```python
from build123d import *

# Parameters (mm, degrees)
ESBO_O2_R                   = 9.5
RESSALTO_EXTRUS_O3_DEPTH    = 9
RESSALTO_EXTRUS_O3_TAPER    = 25
CORTE_EXTRUS_O1_DEPTH       = 8
CORTE_EXTRUS_O4_DEPTH       = 10
CORTE_EXTRUS_O4_DEPTH_BACK  = 8
ESBO_O12_R                  = 1.55
CORTE_EXTRUS_O5_DEPTH       = 5
CORTE_EXTRUS_O5_DEPTH_BACK  = 8
ESBO_O20_R                  = 2.65
CORTE_EXTRUS_O6_DEPTH       = 9.8
CORTE_EXTRUS_O6_DEPTH_BACK  = 10
ESBO_O36_R                  = 1.6
CORTE_EXTRUS_O8_DEPTH       = 10
RESSALTO_EXTRUS_O4_START    = 10
ESBO_O36_3_R                = 9.5
ESBO_O36_3_R_2              = 4
ESBO_O36_3_R_3              = 1.6
RESSALTO_EXTRUS_O4_DEPTH    = 10
CORTE_EXTRUS_O10_DEPTH      = 10
CORTE_EXTRUS_O10_DEPTH_BACK = 9.9
CORTE_EXTRUS_O11_DEPTH      = 9.9
CORTE_EXTRUS_O11_DEPTH_BACK = 9.9


with BuildPart() as part:
    # Esbo_o2 → Ressalto-extrus_o3 (new body)
    with BuildSketch(Plane.XY.offset(10)):
        Circle(ESBO_O2_R)
    extrude(amount=RESSALTO_EXTRUS_O3_DEPTH, taper=RESSALTO_EXTRUS_O3_TAPER)

    # Esbo_o8 → Corte-extrus_o1 (cut)
    with BuildSketch(Plane.XY.offset(19)):
        with BuildLine():
            ThreePointArc((-1.687453703, 1.25), (-1.875499933, -0.944722181), (0, -2.1))
            Line((0, -2.1), (0, 1.25))
            Line((0, 1.25), (-1.687453703, 1.25))
        make_face()
        with BuildLine():
            Line((0, 1.25), (0, -2.1))
            ThreePointArc((0, -2.1), (1.48492424, -1.48492424), (2.1, 0))
            ThreePointArc((2.1, 0), (1.994198182, 0.65815926), (1.687453703, 1.25))
            Line((1.687453703, 1.25), (0, 1.25))
        make_face()
    extrude(amount=-CORTE_EXTRUS_O1_DEPTH, mode=Mode.SUBTRACT)

    # Esbo_o12 → Corte-extrus_o4 (cut, two sides: drawn at the far end of the back side and taken through both)
    with BuildSketch(Plane(origin=(0, 9.25, 0), x_dir=(-1, 0, 0), z_dir=(0, -1, 0)).offset(-CORTE_EXTRUS_O4_DEPTH_BACK)):
        with Locations(Location((0.013800593, -14.999427624, 0), (0, 0, 335.62815521))):
            Circle(ESBO_O12_R)
    extrude(amount=CORTE_EXTRUS_O4_DEPTH + CORTE_EXTRUS_O4_DEPTH_BACK, mode=Mode.SUBTRACT)

    # Esbo_o20 → Corte-extrus_o5 (cut, two sides: drawn at the far end of the back side and taken through both)
    with BuildSketch(Plane(origin=(0, 9.25, 0), x_dir=(-1, 0, 0), z_dir=(0, -1, 0)).offset(-CORTE_EXTRUS_O5_DEPTH_BACK)):
        with Locations(Location((0.013800593, -14.999427624, 0), (0, 0, 10.257774757))):
            Circle(ESBO_O20_R)
    extrude(amount=CORTE_EXTRUS_O5_DEPTH + CORTE_EXTRUS_O5_DEPTH_BACK, mode=Mode.SUBTRACT)

    # Esbo_o25 → Corte-extrus_o6 (cut, two sides: drawn at the far end of the back side and taken through both)
    with BuildSketch(Plane(origin=(0, 0, 20), x_dir=(-1, 0, 0), z_dir=(0, 0, -1)).offset(-CORTE_EXTRUS_O6_DEPTH_BACK)):
        Polygon((7.134775628, 3.121360799), (4.053715986, 2.352982757), (3.178621068, -0.699482185), (5.384585793, -2.983569084), (8.465645436, -2.215191043), (9.340740353, 0.837273899), align=None)
        Polygon((-5.961169976, 3.129376222), (-8.940704294, 2.0313286), (-9.479534318, -1.098047621), (-7.038830024, -3.129376222), (-4.059295706, -2.0313286), (-3.520465682, 1.098047621), align=None)
    extrude(amount=CORTE_EXTRUS_O6_DEPTH + CORTE_EXTRUS_O6_DEPTH_BACK, mode=Mode.SUBTRACT)

    # Esbo_o36 → Corte-extrus_o8 (cut)
    with BuildSketch(Plane(origin=(0, 0, 10), x_dir=(-1, 0, 0), z_dir=(0, 0, -1))):
        with Locations((-6.5, 0)):
            Circle(ESBO_O36_R)
        with Locations((6.5, 0)):
            Circle(ESBO_O36_R)
    extrude(amount=-CORTE_EXTRUS_O8_DEPTH, mode=Mode.SUBTRACT)

    # Esbo_o36_3 → Ressalto-extrus_o4 (add)
    # profile 1 of 2: a face of its own
    with BuildSketch(Plane(origin=(0, 0, 10), x_dir=(-1, 0, 0), z_dir=(0, 0, -1)).offset(RESSALTO_EXTRUS_O4_START)):
        Circle(ESBO_O36_3_R)
        Circle(ESBO_O36_3_R_2, mode=Mode.SUBTRACT)
        with Locations((6.5, 0)):
            Circle(ESBO_O36_3_R_3, mode=Mode.SUBTRACT)
        with Locations((-6.5, 0)):
            Circle(ESBO_O36_3_R_3, mode=Mode.SUBTRACT)
    # profile 2 of 2: a face of its own
    with BuildSketch(Plane(origin=(0, 0, 10), x_dir=(-1, 0, 0), z_dir=(0, 0, -1)).offset(RESSALTO_EXTRUS_O4_START)):
        with BuildLine():
            Line((0.99979998, 0.98), (-0.99979998, 0.98))
            ThreePointArc((-0.99979998, 0.98), (-0.529282546, -1.296094127), (1.4, 0))
            ThreePointArc((1.4, 0), (1.296094127, 0.529282546), (0.99979998, 0.98))
        make_face()
    extrude(amount=-RESSALTO_EXTRUS_O4_DEPTH)

    # Esbo_o49 → Corte-extrus_o10 (cut, two sides: drawn at the far end of the back side and taken through both)
    with BuildSketch(Plane(origin=(0, 0, 20), x_dir=(-1, 0, 0), z_dir=(0, 0, -1)).offset(-CORTE_EXTRUS_O10_DEPTH_BACK)):
        with BuildLine():
            Line((8.371054684, 4.491708302), (4.673014458, 2.507428111))
            Line((4.673014458, 2.507428111), (4.053715986, 2.352982757))
            Line((4.053715986, 2.352982757), (3.178621068, -0.699482185))
            Line((3.178621068, -0.699482185), (4.760398724, -2.337277014))
            Line((4.760398724, -2.337277014), (7.818914356, -5.395792647))
            ThreePointArc((7.818914356, -5.395792647), (9.069996868, -2.825801976), (9.5, 0))
            ThreePointArc((9.5, 0), (9.213441797, 2.31570513), (8.371054684, 4.491708302))
        make_face()
    extrude(amount=CORTE_EXTRUS_O10_DEPTH + CORTE_EXTRUS_O10_DEPTH_BACK, mode=Mode.SUBTRACT)

    # Esbo_o49_4 → Corte-extrus_o11 (cut, two sides: drawn at the far end of the back side and taken through both)
    with BuildSketch(Plane(origin=(0, 0, 20), x_dir=(-1, 0, 0), z_dir=(0, 0, -1)).offset(-CORTE_EXTRUS_O11_DEPTH_BACK)):
        with BuildLine():
            Line((-3.520465682, 1.098047621), (-4.830623712, 2.188454798))
            Line((-4.830623712, 2.188454798), (-8.141518287, 4.89547546))
            ThreePointArc((-8.141518287, 4.89547546), (-9.48963755, 0.443597976), (-8.562700205, -4.114628197))
            Line((-8.562700205, -4.114628197), (-4.779997666, -2.296928855))
            Line((-4.779997666, -2.296928855), (-4.059295706, -2.0313286))
            Line((-4.059295706, -2.0313286), (-3.520465682, 1.098047621))
        make_face()
    extrude(amount=CORTE_EXTRUS_O11_DEPTH + CORTE_EXTRUS_O11_DEPTH_BACK, mode=Mode.SUBTRACT)


solid = part.part
```
Verification items for the finished model (mm, model axes). A direction names the side the tool comes from. Give positions to 0.01 mm unless a question says otherwise; leave off trailing zeros. Write each loop counter-clockwise with the first axis right and the second up, starting at its lowest first coordinate (ties: lowest second). Pieces come first, ordered by that corner, then holes. Notation, with made-up numbers: (49.25, 52.25) - (96.25, 52.25) arc R20 cw to (96.25, 85.25) - close; hole circle Ø10 at (25.5, 12). An arc over 180 degrees is marked (long way). Put each result on its own line as item: value.
Q1. Section check A-A on z = 6. Record the cut outline in (x, y).
Result:
outline: circle Ø19 at (0, 0); (-1, 0.98) arc R1.4 ccw (long way) to (1, 0.98) - close; hole circle Ø3.2 at (-6.5, 0); hole circle Ø8 at (0, 0); hole circle Ø3.2 at (6.5, 0)
Q2. Mould release check, pull along X, two halves, no side actions. Record for faces 6 (the face through (-5.726, 3.073, 12.563)), 7 (the face through (5.85, -2.81, 12.63)), 8 (the face through (-8, -1, 10)), 9 (the face through (8.1, 0.07, 4.98)): released by +X, released by -X, zero draft, split by the parting line, or undercut.
Result:
face 6: released by -X
face 7: released by +X
face 8: zero draft
face 9: undercut
Q3. Scan lines: probe 1 along Y at (x, z) = (0.25, 6.5); probe 2 along X at (y, z) = (-0.25, 8.75); probe 3 along Z at (x, y) = (-2.25, 0.5). Record each from-to range of solid material in increasing order. Write a range as from..to.
Result:
probe 1: -9.5..-3.99, -1.38..0.98, 3.99..9.5
probe 2: -9.5..-8.08, -4.92..-3.99, -1.38..1.38, 3.99..4.92, 8.08..9.5
probe 3: 10..19
Q4. Set-up check for faces 1 (the face through (0.794, 5.895, 12.475)), 2 (the face through (-6.268, -3.845, 12.034)), 3 (the face through (2, 0, 10)), 4 (the face through (8, 1, 10.1)), 5 (the face through (0, 0, 11)): record each of +Z, -Z, +X, -X, +Y, -Y from which the full face is reachable in a straight line by a thin tool's end or side.
Result:
face 1: +Y
face 2: +Z, -X
face 3: -Z
face 4: +Z, +X
face 5: +Z
Q5. Depth check by flat-ended pin: P1, Ø1.6, axis at x = 1, z = 14.5, coming from the +Y side; P2, Ø3, axis at x = -6.5, y = 0, coming from the -Z side; P3, Ø1.7, axis at x = -0.5, z = 16.5, coming from the -Y side; P4, Ø4, axis at x = 7, z = 12.5, coming from the -Y side. Enter the tip coordinate at first touch or a pass-through.
Result:
P1: y = 4.25
P2: through
P3: y = -6.85
P4: y = -7.07
